The listing builds one solid part. Answer for the finished solid, in the listing's coordinates (mm). Face numbers are marked on the shaded views. A direction names the side the tool comes from. Give positions to 0.01 mm unless a question says otherwise; leave off trailing zeros. Order: outer loops, then holes, each group sorted by start corner. A loop starts at its lowest first (then second) coordinate and runs counter-clockwise, first axis right, second up. Notation, with made-up numbers: M 73.25,2 L 84.25,2 A22 ccw 84.25,35 Z; hole C -32.75,-28 d11. An arc over 180 degrees is marked long. Answer as a JSON object with one key per item and string values. Group by question number.
```python
from build123d import *

# Parameters (mm, degrees)
CROQUIS1_R              = 1.016
SALIENTE_EXTRUIR1_DEPTH = 3.1242


with BuildPart() as part:
    # Croquis1 → Saliente-Extruir1 (new body)
    with BuildSketch(Plane.XY):
        with BuildLine():
            Line((-1.7e-08, 9.525), (-3.175, 9.525))
            ThreePointArc((-3.175, 9.525), (-9.910192091, 6.735192091), (-12.7, 0))
            ThreePointArc((-12.7, 0), (-10.952129933, -5.499261314), (-6.35, -8.980256121))
            Line((-6.35, -8.980256121), (-6.35, -3.175))
            Line((-6.35, -3.175), (-6.35, 3.175))
            ThreePointArc((-6.35, 3.175), (-4.490128067, 7.665128054), (-1.7e-08, 9.525))
        make_face()
        with Locations((-9.525, 0)):
            Circle(CROQUIS1_R, mode=Mode.SUBTRACT)
        with BuildLine():
            ThreePointArc((-12.7, 0), (-9.910192091, 6.735192091), (-3.175, 9.525))
            Line((-3.175, 9.525), (-1.7e-08, 9.525))
            Line((-1.7e-08, 9.525), (3.175, 9.525))
            ThreePointArc((3.175, 9.525), (9.910192091, 6.735192091), (12.7, 0))
            ThreePointArc((12.7, 0), (8.980256121, 8.980256121), (0, 12.7))
            ThreePointArc((0, 12.7), (-8.980256121, 8.980256121), (-12.7, 0))
        make_face()
        with BuildLine():
            Line((3.175, 9.525), (-1.7e-08, 9.525))
            ThreePointArc((-1.7e-08, 9.525), (4.490128054, 7.665128067), (6.35, 3.175))
            Line((6.35, 3.175), (6.35, -3.175))
            Line((6.35, -3.175), (6.35, -8.980256121))
            ThreePointArc((6.35, -8.980256121), (10.952129933, -5.499261314), (12.7, 0))
            ThreePointArc((12.7, 0), (9.910192091, 6.735192091), (3.175, 9.525))
        make_face()
        with Locations((9.525, 0)):
            Circle(CROQUIS1_R, mode=Mode.SUBTRACT)
    extrude(amount=SALIENTE_EXTRUIR1_DEPTH)


solid = part.part
```
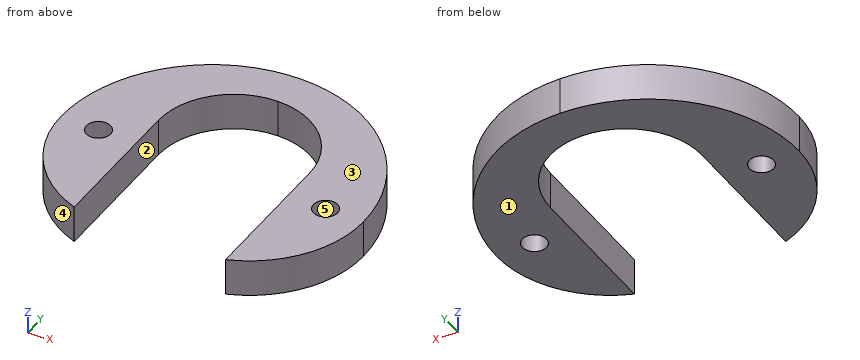
Item 1: Section A-A (z = 2.1) is taken. Determine the outline of the cut face in (x, y) (3 decimals).
Item 2: Flat-ended cylindrical pins translate along their axes: P1, Ø1.6, axis at x = 9.525, y = 0, coming from the +Z side; P2, Ø1, axis at y = 6.5, z = 0.5, coming from the -X side. Find the tip coordinate at first contact, or state that the pin passes through.
Item 3: A tool of negligible diameter and unlimited length cuts with its end or side. For the marked faces 1 and 2, from which of +Z, -Z, +X, -X, +Y, -Y can it reach the whole face along a straight path? Write none if from no direction.
Item 4: Section D-D (x = -2.5) is taken. Determine the outline of the cut face in (y, z).
Item 5: Determine the mould class of the marked faces 3, 4 and 5 for opening direction Y: released by +Y, released by -Y, zero draft, split by the parting line, or undercut.
Item 6: Section B-B (y = -7) is taken. Determine the outline of the cut face in (x, z).
Item 7: Consider probe 1 along X at (y, z) = (-0.5, 0.5); probe 2 along X at (y, z) = (-3.25, 2.05); probe 3 along X at (y, z) = (4, 1.9). Determine where each line is inside the solid, lowest interval first. Write a range as from..to.
Item 8: Section C-C (x = -9) is taken. Determine the outline of the cut face in (y, z), and give its area (3 significant figures).
Values found:
{
 "1": {"outline": "M -12.7,0 A9.525 ccw -6.35,-8.98 L -6.35,3.175 A6.35 cw 6.35,3.175 L 6.35,-8.98 A9.525 ccw 12.7,0 A12.7 ccw Z; hole C -9.525,0 d2.032; hole C 9.525,0 d2.032"},
 "2": {"P1": "passes through", "P2": "stops at x = -11.19"},
 "3": {"face 1": "-Z, +X, -X, +Y, -Y", "face 2": "+Z, -Z, -Y"},
 "4": {"outline": "M 9.01,0 L 12.45,0 L 12.45,3.12 L 9.01,3.12 Z"},
 "5": {"face 3": "zero draft", "face 4": "released by -Y", "face 5": "undercut"},
 "6": {"outline": "M -9.63,0 L -6.35,0 L -6.35,3.12 L -9.63,3.12 Z; M 6.35,0 L 9.63,0 L 9.63,3.12 L 6.35,3.12 Z"},
 "7": {"probe 1": "x = -12.69..-10.41, -8.64..-6.35, 6.35..8.64, 10.41..12.69", "probe 2": "x = -12.13..-6.35, 6.35..12.13", "probe 3": "x = -12.05..-6.3, 6.3..12.05"},
 "8": {"outline": "M -7.54,0 L -0.87,0 L -0.87,3.12 L -7.54,3.12 Z; M 0.87,0 L 8.96,0 L 8.96,3.12 L 0.87,3.12 Z", "area": "46.1 mm^2"}
}
